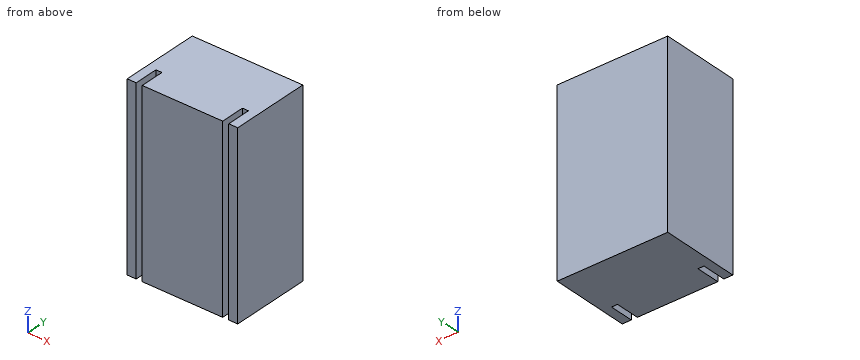
```python
from build123d import *

# Parameters (mm, degrees)
SKIZZE1_W                       = 46
SKIZZE1_H                       = 33
AUFSATZ_LINEAR_AUSTRAGEN1_DEPTH = 75
SKIZZE2_W                       = 2.5
SKIZZE2_H                       = 10
SCHNITT_LINEAR_AUSTRAGEN1_DEPTH = 81.163894616


with BuildPart() as part:
    # Skizze1 → Aufsatz-Linear austragen1 (new body)
    with BuildSketch(Plane.XY):
        Rectangle(SKIZZE1_W, SKIZZE1_H)
    extrude(amount=AUFSATZ_LINEAR_AUSTRAGEN1_DEPTH)

    # Skizze2 → Schnitt-Linear austragen1 (cut, through all)
    with BuildSketch(Plane.XY.offset(75)):
        with Locations((-18, -11.5)):
            Rectangle(SKIZZE2_W, SKIZZE2_H)
        with Locations((18, -11.5)):
            Rectangle(SKIZZE2_W, SKIZZE2_H)
    extrude(amount=-SCHNITT_LINEAR_AUSTRAGEN1_DEPTH, mode=Mode.SUBTRACT)


solid = part.part
```
Can you work these out from the model? Positions are in its coordinate system, mm. Coordinates: 2 decimals unless noted, no trailing zeros. Order: outer loops, then holes, each group sorted by start corner. A loop starts at its lowest first (then second) coordinate and runs counter-clockwise, first axis right, second up.
1. If we section it at A-A (z = 42): Please give me the cut outline in (x, y).
2. If we section it at B-B (x = -18): Please give me the cut outline in (y, z), then the cut area to 4 significant figures.
3. I'm going to push flat-ended pins straight in: pin 1 (4 mm diameter, centred on x = -17, z = 60, fed in from -Y); pin 2 (0.8 mm diameter, centred on x = 18.5, z = 47.5, fed in from -Y). Where does each tip first touch, or does it pass through?
4. I need wall thicknesses on line 1 (X direction, y = -11, z = 49); line 2 (Y direction, x = -17.5, z = 60.5). Which ranges of each line are inside material? Lowest first, please.
Entries:
1. outline: (-23, -16.5) - (-19.25, -16.5) - (-19.25, -6.5) - (-16.75, -6.5) - (-16.75, -16.5) - (16.75, -16.5) - (16.75, -6.5) - (19.25, -6.5) - (19.25, -16.5) - (23, -16.5) - (23, 16.5) - (-23, 16.5) - close
2. outline: (-6.5, 0) - (16.5, 0) - (16.5, 75) - (-6.5, 75) - close
2. area: 1,725 mm2
3. pin 1: stops at y = -16.5
3. pin 2: stops at y = -6.5
4. line 1: x = -23 to -19.25, -16.75 to 16.75, 19.25 to 23
4. line 2: y = -6.5 to 16.5
